Input: part model. Units: mm. Frame: model coordinates. Give positions to 0.01 mm unless a question says otherwise; leave off trailing zeros. Loops run counter-clockwise (first coordinate to the right, second up) from the corner with the lowest first, then second, coordinate; pieces in that order, holes last. Notation, with made-up numbers: M 31.25,38 L 90.25,38 A22 ccw 90.25,48 Z; hole C 25,6 d3. An arc over 180 degrees is marked long. Return JSON: item names as keys, results as strings. Group by question number.
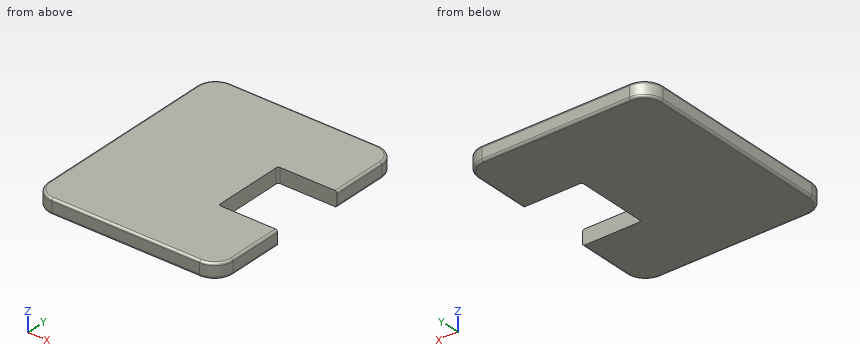
```python
from build123d import *

# Parameters (mm, degrees)
F1_DEPTH = 20
F2_R     = 3
F3_W     = 3
F3_H     = 18
F4_DEPTH = 25
F6_W     = 3
F6_H     = 64
F7_DEPTH = 25


with BuildPart() as f1:
    # F0 (on Top) → F1 (new body)
    with BuildSketch(Plane.XY):
        with BuildLine():
            Line((-100, -150), (100, -150))
            ThreePointArc((100, -150), (117.67767, -142.67767), (125, -125))
            Line((125, -125), (125, 125))
            ThreePointArc((125, 125), (117.67767, 142.67767), (100, 150))
            Line((100, 150), (-100, 150))
            ThreePointArc((-100, 150), (-117.67767, 142.67767), (-125, 125))
            Line((-125, 125), (-125, -125))
            ThreePointArc((-125, -125), (-117.67767, -142.67767), (-100, -150))
        make_face()
    extrude(amount=F1_DEPTH)

    # F2
    f2_edges = [f1.edges().sort_by_distance(p)[0] for p in [
        (-117.67767, -142.67767, 20),
        (0, -150, 20),
        (117.67767, -142.67767, 20),
        (125, 0, 20),
        (117.67767, 142.67767, 20),
        (0, 150, 20),
        (-117.67767, 142.67767, 20),
        (-125, 0, 20),
        (-117.67767, -142.67767, 0),
        (0, -150, 0),
        (117.67767, -142.67767, 0),
        (125, 0, 0),
        (117.67767, 142.67767, 0),
        (0, 150, 0),
        (-117.67767, 142.67767, 0),
        (-125, 0, 0),
    ]]
    fillet(f2_edges, radius=F2_R)

    # F3 (on face) → F4 (cut)
    with BuildSketch(Plane(origin=(0, 0, 0), x_dir=(1, 0, 0), z_dir=(0, 0, -1))):
        with BuildLine():
            Line((122, 32), (122, 50))
            Line((122, 50), (48, 50))
            ThreePointArc((48, 50), (45.87868, 49.12132), (45, 47))
            Line((45, 47), (45, 35))
            ThreePointArc((45, 35), (45.87868, 32.87868), (48, 32))
            Line((48, 32), (122, 32))
        make_face()
        with Locations((123.5, 41)):
            Rectangle(F3_W, F3_H)
        with Locations((123.5, -41)):
            Rectangle(F3_W, F3_H)
        with BuildLine():
            Line((122, -50), (122, -32))
            Line((122, -32), (48, -32))
            ThreePointArc((48, -32), (45.87868, -32.87868), (45, -35))
            Line((45, -35), (45, -47))
            ThreePointArc((45, -47), (45.87868, -49.12132), (48, -50))
            Line((48, -50), (122, -50))
        make_face()
    extrude(amount=-F4_DEPTH, mode=Mode.SUBTRACT)

    # F3 (on face) + F6 (on face) → F7 (cut)
    with BuildSketch(Plane(origin=(0, 0, 0), x_dir=(1, 0, 0), z_dir=(0, 0, -1))):
        with BuildLine():
            Line((122, -32), (122, 32))
            Line((122, 32), (48, 32))
            ThreePointArc((48, 32), (45.87868, 32.87868), (45, 35))
            Line((45, 35), (45, -35))
            ThreePointArc((45, -35), (45.87868, -32.87868), (48, -32))
            Line((48, -32), (122, -32))
        make_face()
    with BuildSketch(Plane(origin=(0, 0, 0), x_dir=(1, 0, 0), z_dir=(0, 0, -1))):
        with Locations((123.5, 0)):
            Rectangle(F6_W, F6_H)
    extrude(amount=-F7_DEPTH, mode=Mode.SUBTRACT)


solid = f1.part
```
Item 1: Section B-B, the plane z = 14. Return loops of the section in (x, y).
Item 2: Section A-A, the plane x = 65.5. Return loops of the section in (y, z).
Item 3: Material intervals for line 1 (Y direction, x = 97.5, z = 16.75); line 2 (Y direction, x = -16, z = 17.5); line 3 (X direction, y = -8, z = 8), sorted ascending. Write a range as from..to.
Item 4: Section C-C, the plane y = 40. Return loops of the section in (x, z), then the cut area to 3 significant figures.
Answer below:
{
 "1": {"outline": "M -125,-125 A25 ccw -100,-150 L 100,-150 A25 ccw 125,-125 L 125,-50 L 48,-50 A3 cw 45,-47 L 45,47 A3 cw 48,50 L 125,50 L 125,125 A25 ccw 100,150 L -100,150 A25 ccw -125,125 Z"},
 "2": {"outline": "M -150,3 A3 ccw -147,0 L -50,0 L -50,20 L -147,20 A3 ccw -150,17 Z; M 50,0 L 147,0 A3 ccw 150,3 L 150,17 A3 ccw 147,20 L 50,20 Z"},
 "3": {"line 1": "-150..-50, 50..150", "line 2": "-149.96..149.96", "line 3": "-125..45"},
 "4": {"outline": "M -125,3 A3 ccw -122,0 L 45,0 L 45,20 L -122,20 A3 ccw -125,17 Z", "area": "3,400 mm^2"}
}
